```python
from build123d import *

# Parameters (mm, degrees)
F0_R     = 1.45
F0_W     = 10
F0_H     = 3
F0_W_2   = 3
F0_H_2   = 10
F1_DEPTH = 3
F2_R     = 1.65
F2_W     = 2.98
F2_H     = 5
F2_W_2   = 39.9
F2_H_2   = 19.4
F3_DEPTH = 25
F2_R_2   = 1.45
F4_DEPTH = 6
F5_W     = 10
F5_H     = 2.98
F6_DEPTH = 12.5


with BuildPart() as f1:
    # F0 (on Right) → F1 (new body)
    with BuildSketch(Plane.YZ):
        Polygon((-35, 50), (-50, 50), (-50, 35), (-47, 35), (-47, 25), (-50, 25), (-50, 5), (-47, 5), (-47, -5), (-50, -5), (-50, -25), (-47, -25), (-47, -35), (-50, -35), (-50, -50), (-35, -50), (-35, -47), (-25, -47), (-25, -50), (-5, -50), (-5, -47), (5, -47), (5, -50), (25, -50), (25, -47), (35, -47), (35, -50), (50, -50), (50, -35), (47, -35), (47, -25), (50, -25), (50, -5), (47, -5), (47, 5), (50, 5), (50, 25), (47, 25), (47, 35), (50, 35), (50, 50), (35, 50), (35, 47), (25, 47), (25, 50), (5, 50), (5, 47), (-5, 47), (-5, 50), (-25, 50), (-25, 47), (-35, 47), align=None)
        with Locations((-8, -20)):
            Circle(F0_R, mode=Mode.SUBTRACT)
        with Locations((-30, 51.5)):
            Rectangle(F0_W, F0_H)
        with Locations((-30, 48.5)):
            Rectangle(F0_W, F0_H)
        with Locations((-48.5, 30)):
            Rectangle(F0_W_2, F0_H_2)
        with Locations((-51.5, 30)):
            Rectangle(F0_W_2, F0_H_2)
        with Locations((0, 51.5)):
            Rectangle(F0_W, F0_H)
        with Locations((0, 48.5)):
            Rectangle(F0_W, F0_H)
        with Locations((-48.5, 0)):
            Rectangle(F0_W_2, F0_H_2)
        with Locations((-51.5, 0)):
            Rectangle(F0_W_2, F0_H_2)
        with Locations((30, 51.5)):
            Rectangle(F0_W, F0_H)
        with Locations((30, 48.5)):
            Rectangle(F0_W, F0_H)
        with Locations((-48.5, -30)):
            Rectangle(F0_W_2, F0_H_2)
        with Locations((-51.5, -30)):
            Rectangle(F0_W_2, F0_H_2)
        with Locations((51.5, 30)):
            Rectangle(F0_W_2, F0_H_2)
        with Locations((48.5, 30)):
            Rectangle(F0_W_2, F0_H_2)
        with Locations((-30, -48.5)):
            Rectangle(F0_W, F0_H)
        with Locations((-30, -51.5)):
            Rectangle(F0_W, F0_H)
        with Locations((51.5, 0)):
            Rectangle(F0_W_2, F0_H_2)
        with Locations((48.5, 0)):
            Rectangle(F0_W_2, F0_H_2)
        with Locations((0, -48.5)):
            Rectangle(F0_W, F0_H)
        with Locations((0, -51.5)):
            Rectangle(F0_W, F0_H)
        with Locations((51.5, -30)):
            Rectangle(F0_W_2, F0_H_2)
        with Locations((48.5, -30)):
            Rectangle(F0_W_2, F0_H_2)
        with Locations((30, -48.5)):
            Rectangle(F0_W, F0_H)
        with Locations((30, -51.5)):
            Rectangle(F0_W, F0_H)
    extrude(amount=F1_DEPTH)

    # F2 (on face) → F3 (cut)
    with BuildSketch(Plane(origin=(0, 0, 0), x_dir=(0, -1, 0), z_dir=(-1, 0, 0))):
        with Locations((-4.05, 29.7)):
            Circle(F2_R)
        with Locations((-4.05, 19.7)):
            Circle(F2_R)
        with Locations((43.95, 29.7)):
            Circle(F2_R)
        with Locations((43.95, 19.7)):
            Circle(F2_R)
        with Locations((11.4694618905, 9.5)):
            Rectangle(F2_W, F2_H)
        with Locations((28.4305381095, 9.5)):
            Rectangle(F2_W, F2_H)
        with Locations((19.95, 24.7)):
            Rectangle(F2_W_2, F2_H_2)
        with Locations((19.95, 39.9)):
            Rectangle(F2_W, F2_H)
    extrude(amount=-F3_DEPTH, mode=Mode.SUBTRACT)

    # F2 (on face) → F4 (join)
    with BuildSketch(Plane(origin=(0, 0, 0), x_dir=(0, -1, 0), z_dir=(-1, 0, 0))):
        Polygon((-50, 50), (-50, 35), (50, 35), (50, 50), (35, 50), (25, 50), (5, 50), (-5, 50), (-25, 50), (-35, 50), align=None)
        with Locations((19.95, 39.9)):
            Rectangle(F2_W, F2_H, mode=Mode.SUBTRACT)
        Polygon((-50, -35), (-50, -50), (-35, -50), (-25, -50), (-5, -50), (5, -50), (25, -50), (35, -50), (50, -50), (-20, 13), (-50, 13), (-50, 5), (-50, -5), (-50, -25), align=None)
        with Locations((8, -20)):
            Circle(F2_R_2, mode=Mode.SUBTRACT)
    extrude(amount=-F4_DEPTH)

    # F5 (on Right) → F6 (cut, symmetric)
    with BuildSketch(Plane.YZ):
        with Locations((-23, -45)):
            Rectangle(F5_W, F5_H)
        with Locations((-8, -35)):
            Rectangle(F5_W, F5_H)
        with Locations((7, -45)):
            Rectangle(F5_W, F5_H)
    extrude(amount=F6_DEPTH, both=True, mode=Mode.SUBTRACT)


solid = f1.part
```
Source: CAD feature listing. Evaluate the final solid. Frame: model axes, mm. A direction names the side the tool comes from. Give positions to 0.01 mm unless a question says otherwise; leave off trailing zeros. Loops run counter-clockwise (first coordinate to the right, second up) from the corner with the lowest first, then second, coordinate; pieces in that order, holes last. Notation, with made-up numbers: (-4.75, 35) - (28.25, 35) arc R10 cw to (28.25, 52) - close; hole circle Ø10 at (-13.75, 8.25). An arc over 180 degrees is marked (long way). Use CSV: the item, a comma, the result in double quotes.
1) Set-up query: faces 1 (the flat face through (1, -25, 51)), 2 (the flat face through (3, 7, -46.49)), 3 (the flat face through (1, -35, 51)), 4 (the flat face through (1, 51, 5)). Return all of +Z, -Z, +X, -X, +Y, -Y with unobstructed straight access to the full face (end or side cutting, diameter ignored); none if empty.
Worked out:
face 1,"+Z, +X, -X"
face 2,"+X, -X"
face 3,"+Z, +X, -X, -Y"
face 4,"+X, -X, +Y"
2) Cut plane C-C (z = 19.7). Output: boundary loops of the cut face in (x, y).
Worked out:
outline,"(0, -50) - (3, -50) - (3, -45.6) - (0, -45.6) - close; (0, -42.3) - (3, -42.3) - (3, -39.9) - (0, -39.9) - close; (0, 0) - (3, 0) - (3, 2.4) - (0, 2.4) - close; (0, 5.7) - (3, 5.7) - (3, 50) - (0, 50) - close"
3) Mould query, pull axis Y, two halves, no side actions, for faces 5 (the cylindrical face through (1.48, -43.59, 28.09)), 6 (the flat face through (1, -53, 0)), 7 (the flat face through (6, 1, 43)). Classes: +Y half, -Y half, draft (parallel to the pull), parting line (faces both ways), or undercut.
Worked out:
face 5,"undercut"
face 6,"-Y half"
face 7,"draft"
4) Cut plane A-A (x = 4.2). Output: boundary loops of the cut face in (y, z).
Worked out:
outline,"(-50, -50) - (50, -50) - (50, 13) - (20, 13) - close; (-50, 35) - (50, 35) - (50, 50) - (-50, 50) - close; hole (-28, -46.49) - (-18, -46.49) - (-18, -43.51) - (-28, -43.51) - close; hole (-21.44, 37.4) - (-18.46, 37.4) - (-18.46, 42.4) - (-21.44, 42.4) - close; hole (-13, -36.49) - (-3, -36.49) - (-3, -33.51) - (-13, -33.51) - close; hole circle Ø2.9 at (-8, -20); hole (2, -46.49) - (12, -46.49) - (12, -43.51) - (2, -43.51) - close"
5) Pin query (flat end, axial travel): P1, Ø0.9, axis at x = 1.5, z = 51, coming from the +Y side; P2, Ø1.5, axis at y = 0, z = -52, coming from the +X side; P3, Ø2.5, axis at x = 1.5, y = -51.5, coming from the +Z side; P4, Ø5, axis at y = 38.5, z = 6.5, coming from the -X side. Return the tip coordinate at first contact, or that it passes through.
Worked out:
P1,"stops at y = 35"
P2,"stops at x = 3"
P3,"stops at z = 35"
P4,"stops at x = 0"
6) Line query: line 1 (Z direction, x = 2.15, y = 4.05); line 2 (Z direction, x = 2.3, y = -19); line 3 (Z direction, x = 4.7, y = 21.5). Output: solid intervals per line, ascending.
Worked out:
line 1,"z = -53 to -46.49, -43.51 to 18.05, 21.35 to 28.05, 31.35 to 53"
line 2,"z = -50 to -46.49, -43.51 to 15, 34.4 to 37.4, 42.4 to 50"
line 3,"z = -50 to 13, 35 to 50"
7) Cut plane B-B (y = -8). Output: boundary loops of the cut face in (x, z).
Worked out:
outline,"(0, -50) - (6, -50) - (6, -36.49) - (0, -36.49) - close; (0, -33.51) - (6, -33.51) - (6, -21.45) - (0, -21.45) - close; (0, -18.55) - (6, -18.55) - (6, -12.2) - (3, -12.2) - (3, 15) - (0, 15) - close; (0, 34.4) - (3, 34.4) - (3, 35) - (6, 35) - (6, 50) - (0, 50) - close"
8) Cut plane D-D (y = 8.5). Output: boundary loops of the cut face in (x, z), and give its area (3 significant figures).
Worked out:
outline,"(0, -50) - (6, -50) - (6, -46.49) - (0, -46.49) - close; (0, -43.51) - (6, -43.51) - (6, 2.65) - (3, 2.65) - (3, 35) - (6, 35) - (6, 50) - (0, 50) - close"
area,"485 mm^2"
